Model file for the job. Use its own axes, mm. Coordinates: 2 decimals unless noted, no trailing zeros. Order: outer loops, then holes, each group sorted by start corner. A loop starts at its lowest first (then second) coordinate and runs counter-clockwise, first axis right, second up. Notation, with made-up numbers: (-32.5, 51.5) -> (16.5, 51.5) arc R20 cw to (16.5, 73.5) -> close; hole circle Ø9 at (-29, 75). An arc over 180 degrees is marked (long way). Write item = value, one per line. Start each with the question number.
Q1. Mould opens along X. For faces 1 (the face through (8.59, 0.04, 1.52)), 2 (the face through (-12.8, 0.5, 3)), 3 (the face through (14.088, 0, 1)) say: +X half, -X half, draft (parallel to the pull), parting line (faces both ways), or undercut.
Q2. Cut at B-B, the plane y = 0. List the corners of the cut face in (x, z).
Q3. Wall check: line 1 (X direction, y = 0.8, z = 2.35); line 2 (Y direction, x = 9.5, z = 0.4); line 3 (X direction, y = 0.4, z = 1.8). Give the ranges that are in metal, low to high. Write a range as from..to.
Q4. Flat gauge pins, fed straight in: pin 1 (1.8 mm diameter, centred on x = -34.41, y = 0, fed in from -Z); pin 2 (2 mm diameter, centred on x = -1.5, y = 1.5, fed in from -Z). Where does each tip first touch, or does it go through?
Q5. Cut at A-A, the plane z = 1.75. List the corners of the cut face in (x, y) (3 decimals), plus the area to 3 significant figures.
from build123d import *

# Parameters (mm, degrees)
SKETCH1_W           = 53
SKETCH1_H           = 4
BOSS_EXTRUDE2_DEPTH = 3
SKETCH3_R           = 1
CUT_EXTRUDE2_DEPTH  = 3
SKETCH4_R           = 0.475
CUT_EXTRUDE3_DEPTH  = 3


with BuildPart() as part:
    # Sketch1 → Boss-Extrude2 (new body)
    with BuildSketch(Plane.XY):
        with Locations((-12.412207578, 0)):
            Rectangle(SKETCH1_W, SKETCH1_H)
    extrude(amount=BOSS_EXTRUDE2_DEPTH)

    # Sketch3 → Cut-Extrude2 (cut)
    with BuildSketch(Plane.XY.offset(3)):
        with Locations((-34.412207578, 0)):
            Circle(SKETCH3_R)
        with Locations((9.587792422, 0)):
            Circle(SKETCH3_R)
    extrude(amount=-CUT_EXTRUDE2_DEPTH, mode=Mode.SUBTRACT)

    # Sketch4 → Cut-Extrude3 (cut)
    with BuildSketch(Plane(origin=(0, 0, 0), x_dir=(-1, 0, 0), z_dir=(0, 0, -1))):
        with Locations((12.412207578, 0)):
            Circle(SKETCH4_R)
    extrude(amount=-CUT_EXTRUDE3_DEPTH, mode=Mode.SUBTRACT)


solid = part.part
Here are the results:
q1.face_1 = undercut
q1.face_2 = draft
q1.face_3 = +X half
q2.outline = (-38.91, 0) -> (-35.41, 0) -> (-35.41, 3) -> (-38.91, 3) -> close; (-33.41, 0) -> (-12.89, 0) -> (-12.89, 3) -> (-33.41, 3) -> close; (-11.94, 0) -> (8.59, 0) -> (8.59, 3) -> (-11.94, 3) -> close; (10.59, 0) -> (14.09, 0) -> (14.09, 3) -> (10.59, 3) -> close
q3.line_1 = -38.91..-35.01, -33.81..8.99, 10.19..14.09
q3.line_2 = -2..-1, 1..2
q3.line_3 = -38.91..-35.33, -33.5..-12.67, -12.16..8.67, 10.5..14.09
q4.pin_1 = through
q4.pin_2 = 0
q5.outline = (-38.912, -2) -> (14.088, -2) -> (14.088, 2) -> (-38.912, 2) -> close; hole circle Ø2 at (-34.412, 0); hole circle Ø0.95 at (-12.412, 0); hole circle Ø2 at (9.588, 0)
q5.area = 205 mm²
